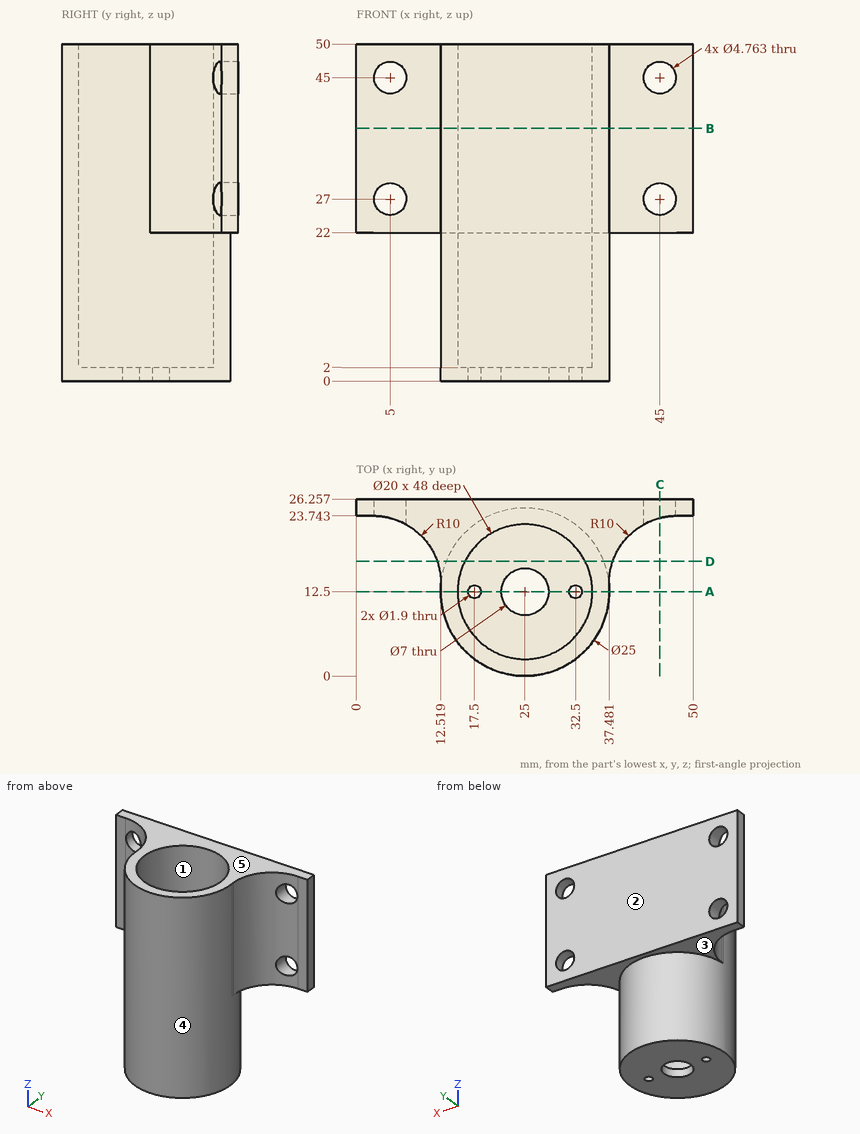
Can you work these out from the drawing? Everything is in mm from the part's minimum corner. A direction names the side the tool comes from. Give positions to 0.01 mm unless a question says otherwise; leave off trailing zeros. Order: outer loops, then holes, each group sorted by start corner. A loop starts at its lowest first (then second) coordinate and runs counter-clockwise, first axis right, second up.
Item 1: If we section it at B-B, the plane z = 37.5: Write out the boundary of the cut face in (x, y).
Item 2: If we section it at D-D, the plane y = 17: Write out the boundary of the cut face in (x, z).
Item 3: I'm going to push flat-ended pins straight in: pin 1 (5.5 mm diameter, centred on x = 45, z = 45, fed in from -Y) (1 decimal); pin 2 (1 mm diameter, centred on x = 16.5, y = 12.5, fed in from +Z); pin 3 (6 mm diameter, centred on x = 5, z = 45, fed in from -Y). Where does each tip first touch, or does it pass through?
Item 4: If we section it at A-A, the plane y = 12.5: Write out the boundary of the cut face in (x, z).
Item 5: If we mould it in two halves opening along Y, with no side actions, what happens to the marked faces 1, 2 and 3? For each: pulls with the +Y half, pulls with the -Y half, needs draft (parallel to the pull), parting line crosses it, or undercut.
Item 6: For the marked faces 4 and 5, which set-ups out of +Z, -Z, +X, -X, +Y, -Y let a thin tool reach every point of the face, with its end or its side?
Item 7: I need wall thicknesses on line 1 (X direction, y = 25, z = 45); line 2 (Z direction, x = 45, y = 24.2); line 3 (Y direction, x = 25, z = 1.15). Which ranges of each line are inside material? Lowest first, please.
Item 8: If we section it at C-C, the plane x = 45: Write out the boundary of the cut face in (y, z).
Values:
1. outline: (0, 23.74) - (2.52, 23.74) arc R10 cw to (12.52, 13.74) - (12.52, 13.19) arc R12.5 ccw (long way) to (37.48, 13.19) - (37.48, 13.74) arc R10 cw to (47.48, 23.74) - (50, 23.74) - (50, 26.26) - (0, 26.26) - close; hole circle Ø20 at (25, 12.5)
2. outline: (11.97, 22) - (13.34, 22) - (13.34, 0) - (36.66, 0) - (36.66, 22) - (38.03, 22) - (38.03, 50) - (33.93, 50) - (33.93, 2) - (16.07, 2) - (16.07, 50) - (11.97, 50) - close
3. pin 1: stops at y = 22.3
3. pin 2: stops at z = 2
3. pin 3: stops at y = 22.11
4. outline: (12.5, 0) - (16.55, 0) - (16.55, 2) - (15, 2) - (15, 50) - (12.5, 50) - close; (18.45, 0) - (21.5, 0) - (21.5, 2) - (18.45, 2) - close; (28.5, 0) - (31.55, 0) - (31.55, 2) - (28.5, 2) - close; (33.45, 0) - (37.5, 0) - (37.5, 50) - (35, 50) - (35, 2) - (33.45, 2) - close
5. face 1: undercut
5. face 2: pulls with the +Y half
5. face 3: needs draft
6. face 4: -Z
6. face 5: +Z, +X, -X, +Y, -Y
7. line 1: x = 0 to 2.62, 7.38 to 42.62, 47.38 to 50
7. line 2: z = 22 to 24.62, 29.38 to 42.62, 47.38 to 50
7. line 3: y = 0 to 9, 16 to 25
8. outline: (23.43, 22) - (26.26, 22) - (26.26, 24.62) - (23.43, 24.62) - close; (23.43, 29.38) - (26.26, 29.38) - (26.26, 42.62) - (23.43, 42.62) - close; (23.43, 47.38) - (26.26, 47.38) - (26.26, 50) - (23.43, 50) - close
